For this review, take the finished solid that the model builds, in its own axes (mm). Give positions to 0.01 mm unless a question says otherwise; leave off trailing zeros. Loops run counter-clockwise (first coordinate to the right, second up) from the corner with the lowest first, then second, coordinate; pieces in that order, holes last.
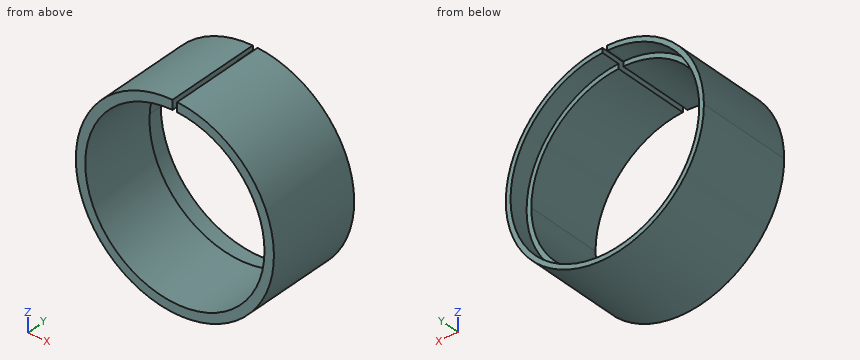
Autodesk Inventor part; units mm, degrees
ref_plane "YZ Plane" through (0, 0, 0) normal (1, 0, 0) x (0, 1, 0)
ref_plane "XZ Plane" through (0, 0, 0) normal (0, 1, 0) x (-1, 0, 0)
ref_plane "XY Plane" through (0, 0, 0) normal (0, 0, 1) x (1, 0, 0)
sketch "スケッチ1" plane through (0, 0, 0) normal (0, 1, 0) x (-1, 0, 0)
  circle A0 centre (0, 0) radius 10
  circle A1 centre (0, 0) radius 10.5
  dimension "d0" = 20
  dimension "d1" = 21
extrude "押し出し1" add sketch "スケッチ1" along normal blind 10
sketch "スケッチ2" plane through (0, 0, 0) normal (0, -1, 0) x (1, 0, 0)
  circle A0 centre (0, 0) radius 9.5
  circle A1 centre (0, 0) radius 10
  dimension "d4" = 19
extrude "押し出し2" add sketch "スケッチ2" against normal blind 8
sketch "スケッチ3" plane through (0, 10, 0) normal (0, 1, 0) x (1, 0, 0)
  line L0 (0.25, -6.9967) -> (0.25, -11.9967)
  line L1 (0.25, -11.9967) -> (-0.25, -11.9967)
  line L2 (-0.25, -11.9967) -> (-0.25, -6.9967)
  line L3 (-0.25, -6.9967) -> (0, -6.9967)
  line L4 (0, -6.9967) -> (0.25, -6.9967)
  circle A0 centre (0, 0) radius 9.5
  point P0 (0.25, -9.4967)
  dimension "d7" = 0.5
  dimension "d10" = 5
extrude "押し出し3" cut sketch "スケッチ3" against normal through all contours L0 A0 L2 L3 L4 | L0 L1 L2 A0 picked at (0.1111, -7.831)
properties part number "zig64"
Q1. Consider section D-D on y = 8.5. Give the boundary of the cut face in (x, z).
Answers:
outline: (-0.25, 10) - (-0.25, 10.5) arc R10.5 ccw (long way) to (0.25, 10.5) - (0.25, 10) arc R10 cw (long way) to start
Q2. For probe 1 along X at (y, z) = (3.5, 0.25); probe 2 along X at (y, z) = (9.5, 0); probe 3 along Z at (x, y) = (0, 8.9), list the stretches that pass through material, from the lowest coordinate up.
Answers:
probe 1: x = -10.5 to -9.5, 9.5 to 10.5
probe 2: x = -10.5 to -10, 10 to 10.5
probe 3: z = -10.5 to -10
Q3. Consider section B-B on x = 1.75. Give the boundary of the cut face in (y, z), plus the area to 3 significant figures.
Answers:
outline: (0, -10.35) - (10, -10.35) - (10, -9.85) - (8, -9.85) - (8, -9.34) - (0, -9.34) - close; (0, 9.34) - (8, 9.34) - (8, 9.85) - (10, 9.85) - (10, 10.35) - (0, 10.35) - close
area: 18.3 mm2
Q4. Consider section C-C on y = 4.75. Give the boundary of the cut face in (x, z), plus the area to 3 significant figures.
Answers:
outline: (-0.25, 9.5) - (-0.25, 10.5) arc R10.5 ccw (long way) to (0.25, 10.5) - (0.25, 9.5) arc R9.5 cw (long way) to start
area: 62.3 mm2
Q5. Consider section A-A on z = -3.75. Give the boundary of the cut face in (x, y).
Answers:
outline: (-9.81, 0) - (-8.73, 0) - (-8.73, 8) - (-9.27, 8) - (-9.27, 10) - (-9.81, 10) - close; (8.73, 0) - (9.81, 0) - (9.81, 10) - (9.27, 10) - (9.27, 8) - (8.73, 8) - close
Q6. For pin 1 Ø1.1 at (y, z) = (6.5, 10) entering from -X; pin 2 Ø4 at (x, y) = (-6, 7) entering from -Z; pin 3 Ø1.5 at (x, y) = (2, 7) entering from -Z, all flat-tipped, find the tip position at first contact; note any pin that passes through.
Answers:
pin 1: stops at x = -4.58
pin 2: stops at z = -9.71
pin 3: stops at z = -10.43
